from build123d import *

# Parameters (mm, degrees)
SKETCH1_W           = 346.7
SKETCH1_H           = 376.55000001
BOSS_EXTRUDE1_DEPTH = 18
SKETCH2_W           = 346.7
SKETCH2_H           = 18
CUT_EXTRUDE1_DEPTH  = 6.35
SKETCH3_W           = 133.35
SKETCH3_H           = 107.95
CUT_EXTRUDE3_DEPTH  = 19
FILLET1_R           = 9.525
SKETCH6_W           = 346.7
SKETCH6_H           = 19.05
CUT_EXTRUDE4_DEPTH  = 6.35
SKETCH7_W           = 346.7
SKETCH7_H           = 12.7
CUT_EXTRUDE5_DEPTH  = 19
FILLET2_R           = 9.525
SKETCH8_R           = 1.7859375
CUT_EXTRUDE6_DEPTH  = 12.65


with BuildPart() as part:
    # Sketch1 → Boss-Extrude1 (new body)
    with BuildSketch(Plane(origin=(0, 0, 0), x_dir=(1, 0, 0), z_dir=(0, 1, 0))):
        with Locations((173.35, -188.275000005)):
            Rectangle(SKETCH1_W, SKETCH1_H)
    extrude(amount=BOSS_EXTRUDE1_DEPTH)

    # Sketch2 → Cut-Extrude1 (cut)
    with BuildSketch(Plane(origin=(0, 18, 0), x_dir=(1, 0, 0), z_dir=(0, 1, 0))):
        with Locations((173.35, -329.45000001)):
            Rectangle(SKETCH2_W, SKETCH2_H)
    extrude(amount=-CUT_EXTRUDE1_DEPTH, mode=Mode.SUBTRACT)

    # Sketch3 → Cut-Extrude3 (cut, through all)
    with BuildSketch(Plane(origin=(0, 18, 0), x_dir=(1, 0, 0), z_dir=(0, 1, 0))):
        with Locations((173.35, -195.57500001)):
            Rectangle(SKETCH3_W, SKETCH3_H)
    extrude(amount=-CUT_EXTRUDE3_DEPTH, mode=Mode.SUBTRACT)

    # Fillet1
    fillet1_edges = [part.edges().sort_by_distance(p)[0] for p in [
        (173.35, 0, 376.55000001),
    ]]
    fillet(fillet1_edges, radius=FILLET1_R)

    # Sketch6 → Cut-Extrude4 (cut)
    with BuildSketch(Plane(origin=(0, 18, 0), x_dir=(1, 0, 0), z_dir=(0, 1, 0))):
        with Locations((173.35, -9.525)):
            Rectangle(SKETCH6_W, SKETCH6_H)
    extrude(amount=-CUT_EXTRUDE4_DEPTH, mode=Mode.SUBTRACT)

    # Sketch7 → Cut-Extrude5 (cut, through all)
    with BuildSketch(Plane(origin=(0, 18, 0), x_dir=(1, 0, 0), z_dir=(0, 1, 0))):
        with Locations((173.35, -370.20000001)):
            Rectangle(SKETCH7_W, SKETCH7_H)
    extrude(amount=-CUT_EXTRUDE5_DEPTH, mode=Mode.SUBTRACT)

    # Fillet2
    fillet2_edges = [part.edges().sort_by_distance(p)[0] for p in [
        (173.35, 0, 363.85000001),
    ]]
    fillet(fillet2_edges, radius=FILLET2_R)

    # Sketch8 → Cut-Extrude6 (cut, through all)
    with BuildSketch(Plane(origin=(0, 11.65, 0), x_dir=(1, 0, 0), z_dir=(0, 1, 0))):
        with Locations((173.35, -9.525)):
            Circle(SKETCH8_R)
        with Locations((173.35, -329.45000001)):
            Circle(SKETCH8_R)
        with Locations((25.4, -329.45000001)):
            Circle(SKETCH8_R)
        with Locations((321.3, -329.45000001)):
            Circle(SKETCH8_R)
        with Locations((321.3, -9.525)):
            Circle(SKETCH8_R)
        with Locations((25.4, -9.525)):
            Circle(SKETCH8_R)
    extrude(amount=-CUT_EXTRUDE6_DEPTH, mode=Mode.SUBTRACT)


solid = part.part
Geometry: final body of the model. Coordinates: model frame, mm. A direction names the side the tool comes from. Give positions to 0.01 mm unless a question says otherwise; leave off trailing zeros. Loops run counter-clockwise (first coordinate to the right, second up) from the corner with the lowest first, then second, coordinate; pieces in that order, holes last. Notation, with made-up numbers: (85.25, 5.25) - (104.25, 5.25) arc R14 cw to (104.25, 32.25) - close; hole circle Ø7 at (-22, 46). An arc over 180 degrees is marked (long way). One line per question, with ' | ' between items. Start each with the question number.
(1) Contact query for flat-ended pins moving along their axis: pin 1 (4 mm diameter, centred on x = 321.3, z = 329.45, fed in from +Y); pin 2 (6 mm diameter, centred on x = 310.5, y = 15.5, fed in from -Z). Output: stop coordinate, or through.
(2) Section query C-C on x = 247. Return loops of the section in (y, z) (3 decimals), then the cut area to 3 significant figures.
(3) Pull-direction query (X, two-part tool) for faces 5 (the flat face through (0, 9, 184)), 6 (the flat face through (240.025, 9, 196)), 7 (the flat face through (171, 0, 135)); classes: released by +X, released by -X, zero draft, split by the parting line, or undercut.
(4) Ray query, line 1 (Z direction, x = 321.3, y = 9); line 2 (Z direction, x = 119, y = 9.75); line 3 (Z direction, x = 25.4, y = 5). Return the intervals inside material, ascending. Write a range as from..to.
(5) Reachability of faces 1 (the flat face through (171, 11.65, 9)), 2 (the flat face through (171, 18, 134)), 3 (the flat face through (172, 9, 141.6)), 4 (the flat face through (171, 11.65, 329)) from +Z, -Z, +X, -X, +Y, -Y: full face, straight path, thin tool, end or side. Return the list, or none.
(6) Section query B-B on y = 14.75. Return loops of the section in (x, z) (3 decimals), then the cut area to 3 significant figures.
(7) Section query A-A on x = 120.5. Return loops of the section in (y, z) (3 decimals).
The answers:
1) pin 1: y = 11.65 | pin 2: z = 19.05
2) outline: (0, 0) - (11.65, 0) - (11.65, 19.05) - (18, 19.05) - (18, 320.45) - (11.65, 320.45) - (11.65, 338.45) - (18, 338.45) - (18, 363.85) - (9.525, 363.85) arc R9.525 ccw to (0, 354.325) - close | area: 6,290 mm2
3) face 5: released by -X | face 6: undercut | face 7: zero draft
4) line 1: 0..7.74, 11.31..327.66, 331.24..363.84 | line 2: 0..141.6, 249.55..363.85 | line 3: 0..7.74, 11.31..327.66, 331.24..362.71
5) face 1: -Z, +X, -X, +Y | face 2: +Z, -Z, +X, -X, +Y | face 3: +Y, -Y | face 4: +X, -X, +Y
6) outline: (0, 19.05) - (346.7, 19.05) - (346.7, 320.45) - (0, 320.45) - close; (0, 338.45) - (346.7, 338.45) - (346.7, 363.85) - (0, 363.85) - close; hole (106.675, 141.6) - (240.025, 141.6) - (240.025, 249.55) - (106.675, 249.55) - close | area: 98,900 mm2
7) outline: (0, 0) - (11.65, 0) - (11.65, 19.05) - (18, 19.05) - (18, 141.6) - (0, 141.6) - close; (0, 249.55) - (18, 249.55) - (18, 320.45) - (11.65, 320.45) - (11.65, 338.45) - (18, 338.45) - (18, 363.85) - (9.525, 363.85) arc R9.525 ccw to (0, 354.325) - close
